Verification items for the finished model (mm, model axes). A direction names the side the tool comes from. Give positions to 0.01 mm unless a question says otherwise; leave off trailing zeros.
(1) Mould release check, pull along Z, two halves, no side actions. Record for faces 4 (the face through (0, 4, -2)), 5 (the face through (0.254, 3.905, 0.867)), 6 (the face through (7.89, -6.083, -6.633)): pulls with the +Z half, pulls with the -Z half, needs draft (parallel to the pull), parting line crosses it, or undercut.
(2) Scan lines: L1, parallel to Y at x = 8.15, z = 0; L2, parallel to X at y = -7, z = 4.25; L3, parallel to Y at x = 8.3, z = 0. Record each from-to range of solid material in increasing order.
(3) Access from +Z, -Z, +X, -X, +Y, -Y to the whole of each face (thin tool, end or side, straight path). Record for faces 1 (the face through (0.5, -3, 2)), 2 (the face through (8, 3, 2)), 3 (the face through (7.5, 6, 0)).
(4) Gauge pin test, flat ends, axial feed: pin 1 (3 mm diameter, centred on x = 6.5, z = 4.5, fed in from +Y); pin 2 (2 mm diameter, centred on x = 5, y = 2, fed in from -Z); pin 3 (1 mm diameter, centred on x = 4.5, z = 4.5, fed in from +Y). Record the tip position at first contact, or that the pin passes through.
```python
from build123d import *
from OCP.BRepFilletAPI import BRepFilletAPI_MakeChamfer

# Parameters (mm, degrees)
CHAMFER1_SIZE      = 0.4
CHAMFER1_SIZE2     = 0.230940108
SKETCH2_R          = 2.5
CUT_EXTRUDE1_DEPTH = 16.305227865
SKETCH3_R          = 4
SKETCH3_R_2        = 3.25
CUT_EXTRUDE2_DEPTH = 0.5
CUT_EXTRUDE3_START = -0.5
SKETCH4_R          = 4
SKETCH4_R_2        = 3.25
CUT_EXTRUDE3_DEPTH = 0.5
CUT_EXTRUDE4_START = -1
CUT_EXTRUDE4_DEPTH = 6.5
CIRPATTERN1_COUNT  = 20


with BuildPart() as part:
    # Sketch1 → Revolve1 (revolve)
    with BuildSketch(Plane.XY, mode=Mode.PRIVATE) as revolve1_sk:
        Polygon((0, 0), (0, 9), (1, 9), (1, 6), (7.5, 6), (7.5, 9), (8.5, 9), (8.5, 0), align=None)
    revolve(revolve1_sk.sketch.rotate(Axis((0, 0, 0), (1, 0, 0)), 90), axis=Axis((0, 0, 0), (1, 0, 0)))

    # Chamfer1: one chamfer whose edges measure the first distance from different faces: ONE call of the kernel's chamfer builder (chamfer() names one face for all edges)
    chamfer1_edges_1 = [part.edges().sort_by_distance(p)[0] for p in [
        (8.5, 0, -9),
    ]]
    chamfer1_side_1 = [part.faces().sort_by_distance(p)[0] for p in [
        (8.5, 0, 0),
    ]]
    chamfer1_edges_2 = [part.edges().sort_by_distance(p)[0] for p in [
        (0, 0, -9),
    ]]
    chamfer1_side_2 = [part.faces().sort_by_distance(p)[0] for p in [
        (0.5, 0, -9),
    ]]
    chamfer1 = BRepFilletAPI_MakeChamfer(part.part.solid().wrapped)
    for e in chamfer1_edges_1:
        chamfer1.Add(CHAMFER1_SIZE, CHAMFER1_SIZE2, e.wrapped, chamfer1_side_1[0].wrapped)  # the first distance lies on this face
    for e in chamfer1_edges_2:
        chamfer1.Add(CHAMFER1_SIZE, CHAMFER1_SIZE2, e.wrapped, chamfer1_side_2[0].wrapped)  # the first distance lies on this face
    add(Compound.cast(chamfer1.Shape()), mode=Mode.REPLACE)

    # Sketch2 → Cut-Extrude1 (cut, through all)
    with BuildSketch(Plane(origin=(8.5, 0, 0), x_dir=(0, 0, -1), z_dir=(1, 0, 0))):
        Circle(SKETCH2_R)
    extrude(amount=-CUT_EXTRUDE1_DEPTH, mode=Mode.SUBTRACT)

    # Sketch3 → Cut-Extrude2 (cut)
    with BuildSketch(Plane(origin=(8.5, 0, 0), x_dir=(0, 0, -1), z_dir=(1, 0, 0))):
        Circle(SKETCH3_R)
        Circle(SKETCH3_R_2, mode=Mode.SUBTRACT)
    extrude(amount=-CUT_EXTRUDE2_DEPTH, mode=Mode.SUBTRACT)

    # Sketch4 → Cut-Extrude3 (cut)
    with BuildSketch(Plane.ZY.offset(CUT_EXTRUDE3_START)):
        with Locations(Location((0, 0, 0), (0, 0, 180))):
            Circle(SKETCH4_R)
        with Locations(Location((0, 0, 0), (0, 0, 180))):
            Circle(SKETCH4_R_2, mode=Mode.SUBTRACT)
    extrude(amount=CUT_EXTRUDE3_DEPTH, mode=Mode.SUBTRACT)

    # Sketch5 → Cut-Extrude4 (cut)
    with BuildSketch(Plane(origin=(8.5, 0, 0), x_dir=(0, 0, -1), z_dir=(1, 0, 0)).offset(CUT_EXTRUDE4_START)):
        with BuildLine():
            Line((-0.399467443, 5.594643379), (-0.447274199, 5.683157544))
            ThreePointArc((-0.447274199, 5.683157544), (-0.654270663, 5.882840909), (-0.93860679, 5.926130044))
            ThreePointArc((-0.93860679, 5.926130044), (0, 6), (0.93860679, 5.926130044))
            ThreePointArc((0.93860679, 5.926130044), (0.654270663, 5.882840909), (0.447274199, 5.683157544))
            Line((0.447274199, 5.683157544), (0.399467443, 5.594643379))
            ThreePointArc((0.399467443, 5.594643379), (0, 5.356388285), (-0.399467443, 5.594643379))
        make_face()
    cut_extrude4 = extrude(amount=-CUT_EXTRUDE4_DEPTH, mode=Mode.SUBTRACT)

    # CirPattern1: Cut-Extrude4 ×20 about axis
    cirpattern1_axis = Axis((0, 0, 0), (1, 0, 0))
    for i in range(1, CIRPATTERN1_COUNT):
        add(cut_extrude4.rotate(cirpattern1_axis, i * 360 / CIRPATTERN1_COUNT), mode=Mode.SUBTRACT)


solid = part.part
```
Ans:
1. face 4: needs draft
1. face 5: undercut
1. face 6: parting line crosses it
2. L1: y = -9 to -4, -3.25 to -2.5, 2.5 to 3.25, 4 to 9
2. L2: x = 0 to 1, 7.5 to 8.5
2. L3: y = -8.95 to -4, -3.25 to -2.5, 2.5 to 3.25, 4 to 8.95
3. face 1: -X
3. face 2: +X
3. face 3: none
4. pin 1: stops at y = 8.34
4. pin 2: stops at z = -5.91
4. pin 3: stops at y = 4.37
